For this review, use the dimensioned drawing (mm, ordinates from the lowest corner) and the shaded views. A direction names the side the tool comes from. Coordinates: 2 decimals unless noted, no trailing zeros. Write each loop counter-clockwise with the first axis right and the second up, starting at its lowest first coordinate (ties: lowest second). Pieces come first, ordered by that corner, then holes. Notation, with made-up numbers: (22, 88.25) - (40, 88.25) arc R28 cw to (40, 124.25) - close; hole circle Ø1 at (77, 13.5). An arc over 180 degrees is marked (long way). Answer as a JSON object with one key per item and string values.
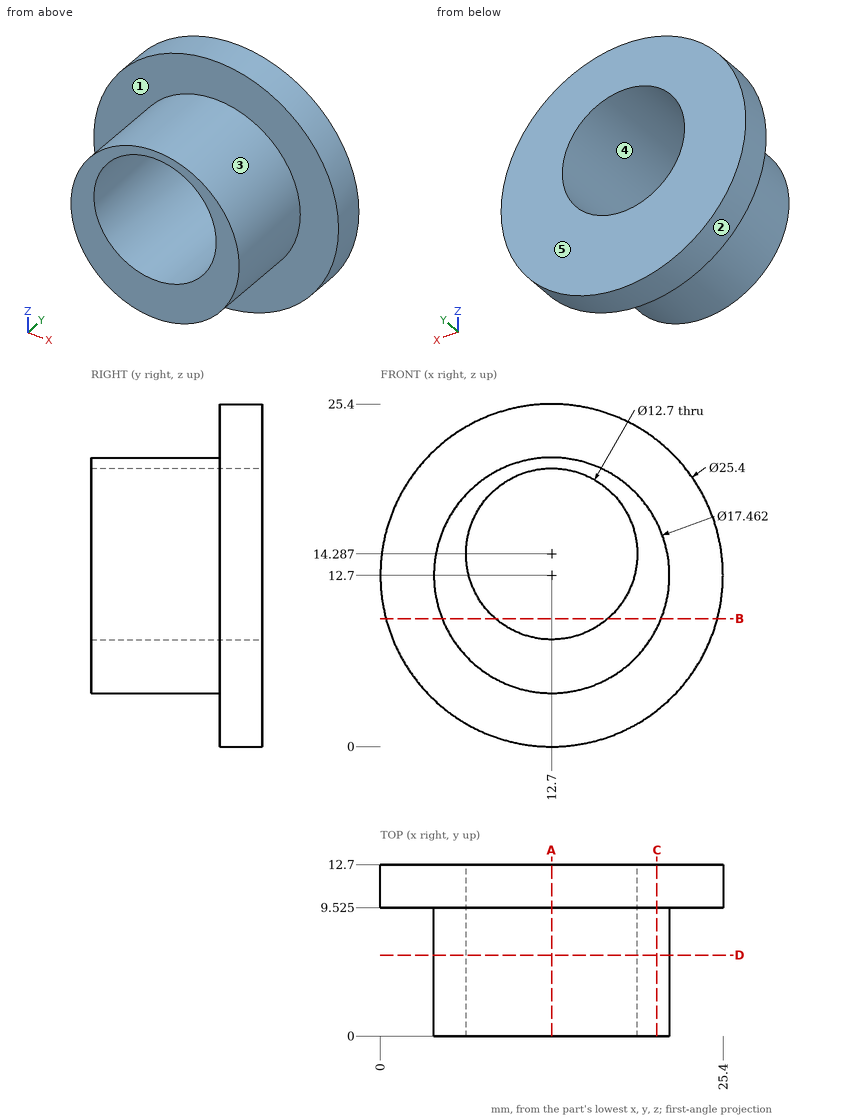
(1) The part is to be moulded in two halves that separate along Z. For the marked faces 3, 4 and 5, say which applies: pulls with the +Z half, pulls with the -Z half, needs draft (parallel to the pull), parting line crosses it, or undercut.
Solved:
{"face 3": "parting line crosses it", "face 4": "undercut", "face 5": "needs draft"}
(2) To check wall thickness, follow line 1 (Z direction, x = 12.7, y = 7.25); line 2 (Y direction, x = 22.5, z = 20.25) (1 decimal); line 3 (X direction, y = 10.5, z = 9.5). State the ranges of each line that lie inside material, in increasing order. Write a range as from..to.
Solved:
{"line 1": "z = 3.97..7.94, 20.64..21.43", "line 2": "y = 9.5..12.7", "line 3": "x = 0.41..8.53, 16.87..24.99"}
(3) Take a section at A-A, the plane x = 12.7. Write out the cut boundary in (y, z) (1 decimal).
Solved:
{"outline": "(0, 4) - (9.5, 4) - (9.5, 0) - (12.7, 0) - (12.7, 7.9) - (0, 7.9) - close; (0, 20.6) - (12.7, 20.6) - (12.7, 25.4) - (9.5, 25.4) - (9.5, 21.4) - (0, 21.4) - close"}
(4) For pin 1 (1 mm diameter, centred on y = 3.5, z = 6.5, fed in from -X) (1 decimal); pin 2 (4 mm diameter, centred on x = 11.5, y = 3.5, fed in from +Z); pin 3 (5 mm diameter, centred on y = 5, z = 14.5, fed in from +X), all flat-tipped, find the tip position at first contact; note any pin that passes through.
Solved:
{"pin 1": "stops at x = 6.1", "pin 2": "stops at z = 21.43", "pin 3": "stops at x = 21.43"}
(5) Take a section at C-C, the plane x = 20.5. Write out the cut boundary in (y, z) (1 decimal).
Solved:
{"outline": "(0, 8.8) - (9.5, 8.8) - (9.5, 2.7) - (12.7, 2.7) - (12.7, 22.7) - (9.5, 22.7) - (9.5, 16.6) - (0, 16.6) - close"}
(6) Take a section at D-D, the plane y = 6. Write out the cut boundary in (x, z).
Solved:
{"outline": "circle Ø17.46 at (12.7, 12.7); hole circle Ø12.7 at (12.7, 14.29)"}
(7) Take a section at B-B, the plane z = 9.5. Write out the cut boundary in (x, y) (1 decimal).
Solved:
{"outline": "(0.4, 9.5) - (4.6, 9.5) - (4.6, 0) - (8.5, 0) - (8.5, 12.7) - (0.4, 12.7) - close; (16.9, 0) - (20.8, 0) - (20.8, 9.5) - (25, 9.5) - (25, 12.7) - (16.9, 12.7) - close"}
(8) Tool access review of the marked faces 1 and 2: name each direction out of +Z, -Z, +X, -X, +Y, -Y from which nothing blocks a thin tool from reaching the whole face with its end or side.
Solved:
{"face 1": "-Y", "face 2": "+Y, -Y"}
